Source: CAD feature listing. Evaluate the final solid. Frame: model axes, mm. A direction names the side the tool comes from. Round coordinates to 2 decimals unless told otherwise and drop trailing zeros. Loops run counter-clockwise (first coordinate to the right, second up) from the corner with the lowest first, then second, coordinate; pieces in that order, holes last. Notation, with made-up numbers: M 41.5,-19 L 87.5,-19 A4 cw 87.5,-14 Z; hole C 31,87.25 d8. An arc over 180 degrees is marked long. Answer as a JSON object with one key per item and string values.
from build123d import *

# Parameters (mm, degrees)
SKETCH_1_R      = 1.55
EXTRUDE_1_DEPTH = 3
FILLET_1_R      = 2
FILLET_2_R      = 0.5


with BuildPart() as part:
    # 草图1 → 凸台-拉伸1 (new body)
    with BuildSketch(Plane(origin=(0, 0, 0), x_dir=(1, 0, 0), z_dir=(0, 1, 0))):
        Polygon((30, -85), (20, -85), (14.705882353, -70), (-16.222232293, -70), (-21.51634994, -85), (-30, -85), (-30, -69.976869686), (-20, -41.643536352), (-20, 41.643536352), (-30, 69.976869686), (-30, 85), (-21.51634994, 85), (-16.222232293, 70), (14.705882353, 70), (20, 85), (30, 85), (30, 69.976869686), (20, 41.643536352), (20, -41.643536352), (30, -69.976869686), align=None)
        with Locations(Location((-25, 75, 0), (0, 0, 270))):
            Circle(SKETCH_1_R, mode=Mode.SUBTRACT)
        with Locations(Location((25, 75, 0), (0, 0, 270))):
            Circle(SKETCH_1_R, mode=Mode.SUBTRACT)
        with Locations(Location((25, -75, 0), (0, 0, 90))):
            Circle(SKETCH_1_R, mode=Mode.SUBTRACT)
        with Locations(Location((-25, -75, 0), (0, 0, 90))):
            Circle(SKETCH_1_R, mode=Mode.SUBTRACT)
        with BuildLine():
            Line((-10.97228498, 0), (0, -11.072893133))
            Line((0, -11.072893133), (10.97228498, 0))
            ThreePointArc((10.97228498, 0), (10.2971634, 10.452899726), (0, 8.532658143))
            ThreePointArc((0, 8.532658143), (-10.2971634, 10.452899726), (-10.97228498, 0))
        make_face(mode=Mode.SUBTRACT)
        Polygon((12.634504731, 65), (0, 44.995367509), (-12.634504731, 65), align=None, mode=Mode.SUBTRACT)
        Polygon((-12.634504731, 17.5), (0, 37.504632491), (12.634504731, 17.5), align=None, mode=Mode.SUBTRACT)
        Polygon((-15, 61.254632491), (-2.365495269, 41.25), (-15, 21.245367509), align=None, mode=Mode.SUBTRACT)
        Polygon((15, 61.254632491), (15, 21.245367509), (2.365495269, 41.25), align=None, mode=Mode.SUBTRACT)
        Polygon((2.365495269, -41.25), (15, -61.254632491), (15, -21.245367509), align=None, mode=Mode.SUBTRACT)
        Polygon((-12.634504731, -65), (12.634504731, -65), (0, -44.995367509), align=None, mode=Mode.SUBTRACT)
        Polygon((-15, -21.245367509), (-15, -61.254632491), (-2.365495269, -41.25), align=None, mode=Mode.SUBTRACT)
        Polygon((12.634504731, -17.5), (-12.634504731, -17.5), (0, -37.504632491), align=None, mode=Mode.SUBTRACT)
    extrude(amount=EXTRUDE_1_DEPTH)

    # 圆角1
    fillet_1_edges = [part.edges().sort_by_distance(p)[0] for p in [
        (-15, 1.5, -21.245367509),
        (-2.365495269, 1.5, -41.25),
        (-15, 1.5, -61.254632491),
        (-12.634504731, 1.5, -17.5),
        (12.634504731, 1.5, -17.5),
        (0, 1.5, -37.504632491),
        (0, 1.5, 44.995367509),
        (-12.634504731, 1.5, 65),
        (12.634504731, 1.5, 65),
        (-2.365495269, 1.5, 41.25),
        (-15, 1.5, 21.245367509),
        (-15, 1.5, 61.254632491),
        (0, 1.5, 37.504632491),
        (12.634504731, 1.5, 17.5),
        (-12.634504731, 1.5, 17.5),
        (-21.51634994, 1.5, -85),
        (-16.222232293, 1.5, -70),
        (14.705882353, 1.5, -70),
        (20, 1.5, -85),
        (30, 1.5, -85),
        (30, 1.5, -69.976869686),
        (20, 1.5, -41.643536352),
        (20, 1.5, 41.643536352),
        (30, 1.5, 69.976869686),
        (30, 1.5, 85),
        (20, 1.5, 85),
        (14.705882353, 1.5, 70),
        (-16.222232293, 1.5, 70),
        (-21.51634994, 1.5, 85),
        (-30, 1.5, 85),
        (-30, 1.5, 69.976869686),
        (-20, 1.5, 41.643536352),
        (-20, 1.5, -41.643536352),
        (-30, 1.5, -69.976869686),
        (-30, 1.5, -85),
        (15, 1.5, 21.245367509),
        (2.365495269, 1.5, 41.25),
        (15, 1.5, 61.254632491),
        (15, 1.5, -61.254632491),
        (2.365495269, 1.5, -41.25),
        (15, 1.5, -21.245367509),
        (-12.634504731, 1.5, -65),
        (0, 1.5, -44.995367509),
        (12.634504731, 1.5, -65),
    ]]
    fillet(fillet_1_edges, radius=FILLET_1_R)

    # 圆角2
    fillet_2_edges = [part.edges().sort_by_distance(p)[0] for p in [
        (0, 1.5, -8.532658143),
    ]]
    fillet(fillet_2_edges, radius=FILLET_2_R)


solid = part.part
Item 1: Section A-A on x = 6. Give the number of separate pieces and of enclosed holes in the cut face, then the cut area to 3 significant figures.
Answer sheet:
{"separate pieces": "8", "enclosed holes": "0", "area": "174 mm²"}
Item 2: Pull-direction query (X, two-part tool) for faces 1 (the flat face through (-26, 1, -85)), 2 (the flat face through (-30, 1, 77)), 3 (the flat face through (15, 1, 41)); classes: pulls with the +X half, pulls with the -X half, needs draft (parallel to the pull), parting line crosses it, or undercut.
Answer sheet:
{"face 1": "needs draft", "face 2": "pulls with the -X half", "face 3": "undercut"}
Item 3: Line query: probe 1 along X at (y, z) = (0.7, 39); probe 2 along X at (y, z) = (0.75, -75); probe 3 along X at (y, z) = (1.45, 51). Output: solid intervals per line, ascending. Write a range as from..to.
Answer sheet:
{"probe 1": "x = -20..-15, -3.79..3.79, 15..20", "probe 2": "x = -30..-26.55, -23.45..-17.99, 16.47..23.45, 26.55..30", "probe 3": "x = -23.3..-15, -8.52..-3.79, 3.79..8.52, 15..23.3"}
Item 4: Access query for faces 4 (the flat face through (-30, 1, -77)), 5 (the flat face through (30, 1, 77)), 6 (the flat face through (0, 1, -65)), 7 (the flat face through (-1, 1, -70)), 8 (the flat face through (-1, 1, 70)). Directions: +Z, -Z, +X, -X, +Y, -Y. A direction counts if a zero-diameter tool reaches every point of the face in a straight line with its end or side. Return the directions, or none.
Answer sheet:
{"face 4": "+Z, -Z, -X, +Y, -Y", "face 5": "+Z, -Z, +X, +Y, -Y", "face 6": "+Y, -Y", "face 7": "-Z, +Y, -Y", "face 8": "+Z, +Y, -Y"}
Item 5: Section C-C on x = -25. Return the cut outline in (y, z), then the cut area to 3 significant figures.
Answer sheet:
{"outline": "M 0,-85 L 3,-85 L 3,-76.55 L 0,-76.55 Z; M 0,-73.45 L 3,-73.45 L 3,-55.81 L 0,-55.81 Z; M 0,55.81 L 3,55.81 L 3,73.45 L 0,73.45 Z; M 0,76.55 L 3,76.55 L 3,85 L 0,85 Z", "area": "157 mm²"}
Item 6: Contact query for flat-ended pins moving along their axis: pin 1 Ø1.5 at (y, z) = (1.5, -6) entering from +X; pin 2 Ø0.9 at (x, y) = (4, 1.5) entering from +Z; pin 3 Ø0.9 at (y, z) = (1, 43.5) entering from +X. Output: stop coordinate, or through.
Answer sheet:
{"pin 1": "stops at x = 20", "pin 2": "stops at z = 70", "pin 3": "stops at x = 20.81"}
Item 7: Section B-B on z = -52. Return the cut outline in (x, y).
Answer sheet:
{"outline": "M -23.66,0 L -15,0 L -15,3 L -23.66,3 Z; M -9.15,0 L -4.42,0 L -4.42,3 L -9.15,3 Z; M 4.42,0 L 9.15,0 L 9.15,3 L 4.42,3 Z; M 15,0 L 23.66,0 L 23.66,3 L 15,3 Z"}
